Input: part model. Units: mm. Frame: model coordinates. A direction names the side the tool comes from. Coordinates: 2 decimals unless noted, no trailing zeros. Order: outer loops, then holes, each group sorted by start corner. A loop starts at its lowest first (then second) coordinate and runs counter-clockwise, first axis right, second up. Notation, with made-up numbers: (89.25, -22.5) -> (122.25, -22.5) arc R20 ccw to (122.25, -0.5) -> close; hole circle Ø8 at (89.5, 30). An arc over 180 degrees is marked (long way). Write each question's results on one line, items separated by ' | '.
```python
from build123d import *

# Parameters (mm, degrees)
SKETCH3_R               = 21
BOSS_EXTRUDE3_DEPTH     = 32
CUT_EXTRUDE1_START      = -30
SKETCH4_R               = 21
SKETCH4_R_2             = 19.31273959
CUT_EXTRUDE1_DEPTH      = 28
SKETCH8_R               = 6.075
SKETCH8_R_2             = 2.409749928
CUT_EXTRUDE2_DEPTH      = 44.657759906
FILLET1_R               = 1
FILLET3_R               = 5
BOSS_EXTRUDE4_START     = -17
SKETCH11_R              = 8
BOSS_EXTRUDE4_DEPTH     = 15
SKETCH12_W              = 6.25
SKETCH12_H              = 3.5
BOSS_EXTRUDE5_DEPTH     = 17
SKETCH15_OUTSIDE_W      = 57.494
SKETCH15_OUTSIDE_H      = 57.494
SKETCH15_OUTSIDE_R      = 21
CUT_EXTRUDE3_DEPTH      = 17
SKETCH16_R              = 25.999161841
SKETCH16_R_2            = 10.063122469
CUT_EXTRUDE4_DEPTH      = 44.657759954
CUT_EXTRUDE5_DEPTH      = 35.948058737
CUT_EXTRUDE5_DEPTH_BACK = 35.948058737
SKETCH17_W              = 34.125667019
SKETCH17_H              = 28.204609122


with BuildPart() as part:
    # Sketch3 → Boss-Extrude3 (new body)
    with BuildSketch(Plane.XY):
        Circle(SKETCH3_R)
    extrude(amount=BOSS_EXTRUDE3_DEPTH)

    # Sketch4 → Cut-Extrude1 (cut)
    with BuildSketch(Plane.XY.offset(32).offset(CUT_EXTRUDE1_START)):
        Circle(SKETCH4_R)
        Circle(SKETCH4_R_2, mode=Mode.SUBTRACT)
    extrude(amount=CUT_EXTRUDE1_DEPTH, mode=Mode.SUBTRACT)

    # Cut-Sweep1: sweep along a curve in space
    with BuildLine() as cut_sweep1_path:
        ThreePointArc((19.31273959, 0, 2), (13.656169127, 13.656169127, 2), (0, 19.31273959, 2))
        ThreePointArc((0, 19.31273959, 2), (-13.656169127, 13.656169127, 2), (-19.31273959, 0, 2))
        ThreePointArc((-19.31273959, 0, 2), (-13.656169127, -13.656169127, 2), (0, -19.31273959, 2))
        ThreePointArc((0, -19.31273959, 2), (13.656169127, -13.656169127, 2), (19.31273959, 0, 2))
    # Sketch7 → Cut-Sweep1 (sweep, cut)
    with BuildSketch(Plane(origin=(0, 0, 0), x_dir=(1, 0, 0), z_dir=(0, 1, 0))):
        with BuildLine():
            Line((-19.31273959, -2), (-19.31273959, -30))
            ThreePointArc((-19.31273959, -30), (-17.146485403, -16), (-19.31273959, -2))
        make_face()
    sweep(path=cut_sweep1_path.line, mode=Mode.SUBTRACT)

    # Sketch8 → Cut-Extrude2 (cut, through all)
    with BuildSketch(Plane(origin=(0, 0, 0), x_dir=(-1, 0, 0), z_dir=(0, 0, -1))):
        Circle(SKETCH8_R)
        with Locations((9.076330186, 5.279334971)):
            Circle(SKETCH8_R_2)
        with Locations((-0.033873107, 10.5)):
            Circle(SKETCH8_R_2)
        with Locations((9.110203293, -5.220665029)):
            Circle(SKETCH8_R_2)
        with Locations((0.033873107, -10.5)):
            Circle(SKETCH8_R_2)
        with Locations((-9.076330186, -5.279334971)):
            Circle(SKETCH8_R_2)
        with Locations((-9.110203293, 5.220665029)):
            Circle(SKETCH8_R_2)
    extrude(amount=-CUT_EXTRUDE2_DEPTH, mode=Mode.SUBTRACT)

    # Sketch10 → Cut-Revolve1 (revolve, cut)
    with BuildSketch(Plane(origin=(0, 0, 0), x_dir=(1, 0, 0), z_dir=(0, 1, 0))):
        Polygon((-6.075, 0), (-15.24176478, -2.795793959), (-19.075, 0), align=None)
    revolve(axis=Axis((0, 0, 2), (0, 0, 1)), mode=Mode.SUBTRACT)

    # Fillet1
    fillet1_edges = [part.edges().sort_by_distance(p)[0] for p in [
        (-21, 0, 2),
        (-21, 0, 30),
    ]]
    fillet(fillet1_edges, radius=FILLET1_R)

    # Fillet3
    # the kernel refuses this fillet: 5 mm, written as the material it adds along each edge
    with BuildSketch(Plane(origin=(0, 0, 2.795793959), x_dir=(-1, 0, 0), z_dir=(0, 1, 0))) as fillet3_piece_1_section:
        with BuildLine():
            CenterArc((15.24176478 - FILLET3_R * 0.185863598659, -FILLET3_R * 1.10216314652), FILLET3_R, 53.894625959, 53.066683648)
            Line((15.24176478 - FILLET3_R * 0.47758946832, -FILLET3_R * 0.145661177375), (15.24176478, 0))
            Line((15.24176478, 0), (15.24176478 + FILLET3_R * 0.403408541274, -FILLET3_R * 0.294228529669))
        make_face()
    fillet3_piece_1 = revolve(axis=Axis((0, 0, 2.795793959), (0, 0, 1)), mode=Mode.PRIVATE)
    fillet3_piece_1 = fillet3_piece_1 - Plane(origin=(-9.110203293, -5.220665029, 2.265856679), x_dir=(-1, 0, 0), z_dir=(0, 0, -1)) * Cylinder(2.409749928, 70, mode=Mode.PRIVATE)
    fillet3_piece_1 = fillet3_piece_1 - Plane(origin=(-0.033873107, -10.5, 2.265856679), x_dir=(-1, 0, 0), z_dir=(0, 0, -1)) * Cylinder(2.409749928, 70, mode=Mode.PRIVATE)
    fillet3_piece_1 = fillet3_piece_1 - Plane(origin=(9.076330186, -5.279334971, 2.265856679), x_dir=(-1, 0, 0), z_dir=(0, 0, -1)) * Cylinder(2.409749928, 70, mode=Mode.PRIVATE)
    fillet3_piece_1 = fillet3_piece_1 - Plane(origin=(9.110203293, 5.220665029, 2.265856679), x_dir=(-1, 0, 0), z_dir=(0, 0, -1)) * Cylinder(2.409749928, 70, mode=Mode.PRIVATE)
    fillet3_piece_1 = fillet3_piece_1 - Plane(origin=(-9.076330186, 5.279334971, 2.265856679), x_dir=(-1, 0, 0), z_dir=(0, 0, -1)) * Cylinder(2.409749928, 70, mode=Mode.PRIVATE)
    fillet3_piece_1 = fillet3_piece_1 - Plane(origin=(0.033873107, 10.5, 2.265856679), x_dir=(-1, 0, 0), z_dir=(0, 0, -1)) * Cylinder(2.409749928, 70, mode=Mode.PRIVATE)
    add(fillet3_piece_1)

    # Sketch11 → Boss-Extrude4 (add)
    with BuildSketch(Plane.XY.offset(32).offset(BOSS_EXTRUDE4_START)):
        Circle(SKETCH11_R)
    extrude(amount=-BOSS_EXTRUDE4_DEPTH)

    # Sketch12 → Boss-Extrude5 (add)
    with BuildSketch(Plane.XY.offset(32)):
        with Locations((-6.125, 0)):
            Rectangle(SKETCH12_W, SKETCH12_H)
        with Locations((6.125, 0)):
            Rectangle(SKETCH12_W, SKETCH12_H)
    extrude(amount=-BOSS_EXTRUDE5_DEPTH)

    # Sketch15 outside → Cut-Extrude3 (cut)
    # profile 1 of 2: a face of its own
    with BuildSketch(Plane.XY.offset(32)):
        Rectangle(SKETCH15_OUTSIDE_W, SKETCH15_OUTSIDE_H)
        Circle(SKETCH15_OUTSIDE_R, mode=Mode.SUBTRACT)
    # profile 2 of 2: a face of its own
    with BuildSketch(Plane.XY.offset(32)):
        with BuildLine():
            Line((-6.207908263, 1.45), (-3.3, 1.45))
            Line((-3.3, 1.45), (-3.3, -1.45))
            Line((-3.3, -1.45), (-6.207908263, -1.45))
            ThreePointArc((-6.207908263, -1.45), (0, -6.375), (6.207908263, -1.45))
            Line((6.207908263, -1.45), (3.3, -1.45))
            Line((3.3, -1.45), (3.3, 1.45))
            Line((3.3, 1.45), (6.207908263, 1.45))
            ThreePointArc((6.207908263, 1.45), (0, 6.375), (-6.207908263, 1.45))
        make_face()
    extrude(amount=-CUT_EXTRUDE3_DEPTH, mode=Mode.SUBTRACT)

    # Sketch16 → Cut-Extrude4 (cut, through all)
    with BuildSketch(Plane.XY.offset(32)):
        Circle(SKETCH16_R)
        Circle(SKETCH16_R_2, mode=Mode.SUBTRACT)
    extrude(amount=-CUT_EXTRUDE4_DEPTH, mode=Mode.SUBTRACT)

    # Sketch17 → Cut-Extrude5 (cut, two sides: drawn at the far end of the back side and taken through both)
    with BuildSketch(Plane(origin=(0, 0, 0), x_dir=(1, 0, 0), z_dir=(0, 1, 0)).offset(-CUT_EXTRUDE5_DEPTH_BACK)):
        with Locations((1.878185032, -13.325973853)):
            Rectangle(SKETCH17_W, SKETCH17_H)
    extrude(amount=CUT_EXTRUDE5_DEPTH + CUT_EXTRUDE5_DEPTH_BACK, mode=Mode.SUBTRACT)


solid = part.part
```
(1) Cut plane D-D, the plane x = -5.5. Return loops of the section in (y, z), plus the area to 3 significant figures.
Return value:
outline: (-8.43, 27.43) -> (-3.22, 27.43) -> (-3.22, 32) -> (-8.43, 32) -> close; (-1.45, 27.43) -> (1.45, 27.43) -> (1.45, 32) -> (-1.45, 32) -> close; (3.22, 27.43) -> (8.43, 27.43) -> (8.43, 32) -> (3.22, 32) -> close | area: 60.8 mm2
(2) Cut plane C-C, the plane x = -0.5. Return loops of the section in (y, z), plus the area to 3 significant figures.
Return value:
outline: (-8.14, 27.43) -> (-6.36, 27.43) -> (-6.36, 32) -> (-8.14, 32) -> close; (6.36, 27.43) -> (8.15, 27.43) -> (8.15, 32) -> (6.36, 32) -> close | area: 16.3 mm2
(3) Reachability of faces 4 (the face through (0.07, 8.09, 29.68)), 5 (the face through (5, 1.45, 30)) from +Z, -Z, +X, -X, +Y, -Y: full face, straight path, thin tool, end or side. Return the list, or none.
Return value:
face 4: +Z, -Z, +Y | face 5: +Z, -Z
(4) Pin query (flat end, axial travel): P1, Ø2, axis at x = -1.5, y = -3.5, coming from the +Z side; P2, Ø1.5, axis at x = 4.5, z = 29.5, coming from the +Y side; P3, Ø1, axis at x = 0.5, z = 28.5, coming from the -Y side; P4, Ø2, axis at x = 0.5, z = 31, coming from the -Y side. Return the tip coordinate at first contact, or that it passes through.
Return value:
P1: through | P2: y = 9.34 | P3: y = -8.32 | P4: y = -8.64
(5) Line query: line 1 along Y through (x, z) = (5.75, 30.5); line 2 along Y through (x, z) = (-5, 28.8); line 3 along X through (y, z) = (-4, 30.2). Output: solid intervals per line, ascending. Write a range as from..to.
Return value:
line 1: -8.26..-2.75, -1.45..1.45, 2.75..8.26 | line 2: -8.73..-3.95, -1.45..1.45, 3.95..8.73 | line 3: -7.03..-4.96, 4.96..7.03
(6) Mould query, pull axis Y, two halves, no side actions, for faces 1 (the face through (5, -1.45, 30)), 2 (the face through (4.97, -8.75, 29.75)), 3 (the face through (5.095, 8.678, 29.746)). Classes: +Y half, -Y half, draft (parallel to the pull), parting line (faces both ways), or undercut.
Return value:
face 1: undercut | face 2: -Y half | face 3: +Y half
(7) Cut plane B-B, the plane y = -5. Return loops of the section in (x, z).
Return value:
outline: (-6.71, 27.43) -> (-3.95, 27.43) -> (-3.95, 32) -> (-6.71, 32) -> close; (3.95, 27.43) -> (6.68, 27.43) -> (6.68, 32) -> (3.95, 32) -> close
